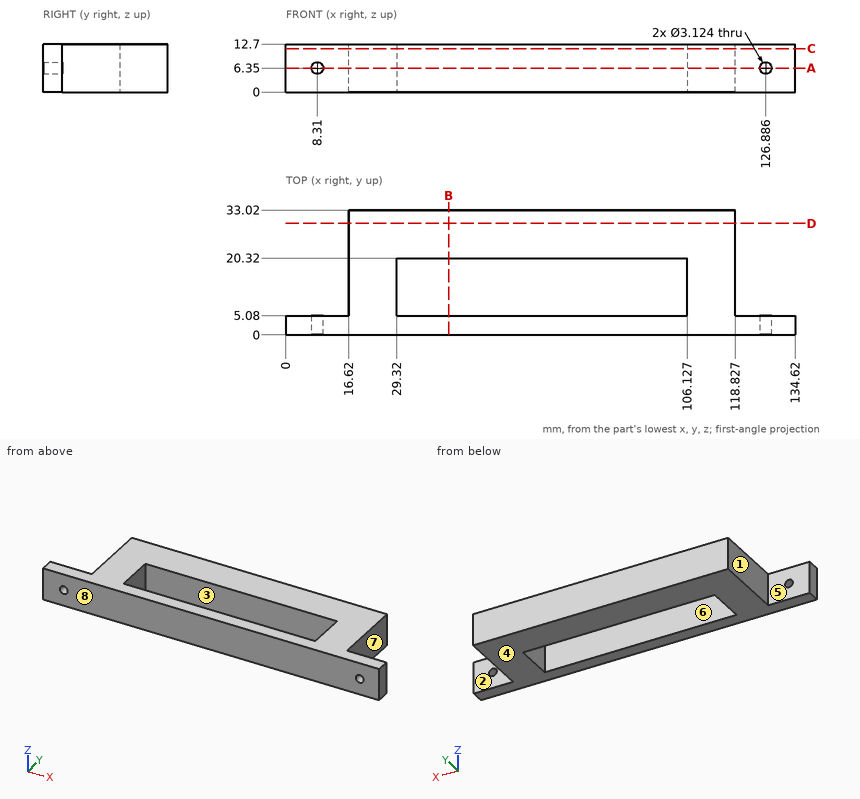
The figure shows three views and two pictorial views of one solid part (mm, origin at its lowest corner). Answer the questions. A direction names the side the tool comes from. Give positions to 0.01 mm unless a question says otherwise; leave off trailing zeros. Write each loop counter-clockwise with the first axis right and the second up, starting at its lowest first coordinate (ties: lowest second). Pieces come first, ordered by that corner, then holes. Notation, with made-up numbers: (69.5, 39.25) - (117.5, 39.25) arc R36 cw to (117.5, 75.25) - close; hole circle Ø2 at (-3.75, 76.25). An arc over 180 degrees is marked (long way). Return JSON: item names as keys, results as strings.
Q1. Consider line 1 along Y through (x, z) = (80.5, 10); line 2 along X through (y, z) = (7, 4.25); line 3 along X through (y, z) = (28.5, 4.5). Determine where each line is inside the solid, lowest interval first. Write a range as [from, to].
Reply:
{"line 1": "[0, 5.08], [20.32, 33.02]", "line 2": "[16.62, 29.32], [106.13, 118.83]", "line 3": "[16.62, 118.83]"}
Q2. A cutting plane is placed at D-D, the plane y = 29.5. Determine the outline of the cut face in (x, z), and give its area (3 significant figures).
Reply:
{"outline": "(16.62, 0) - (118.83, 0) - (118.83, 12.7) - (16.62, 12.7) - close", "area": "1,300 mm²"}
Q3. Given P1, Ø5, axis at y = 26, z = 2, coming from the +X side; P2, Ø1.9, axis at x = 126.89, z = 6.35, coming from the -Y side, each flat-ended and moving along its own axis, determine where each tip first touches the part or whether it passes through.
Reply:
{"P1": "x = 118.83", "P2": "through"}
Q4. A cutting plane is placed at B-B, the plane x = 43. Determine the outline of the cut face in (y, z).
Reply:
{"outline": "(0, 0) - (5.08, 0) - (5.08, 12.7) - (0, 12.7) - close; (20.32, 0) - (33.02, 0) - (33.02, 12.7) - (20.32, 12.7) - close"}
Q5. For the marked faces 1, 2, 3 and 4, determine the directions among +Z, -Z, +X, -X, +Y, -Y from which every point of the face is accessible in a straight line to the end or side of a thin tool.
Reply:
{"face 1": "+Z, -Z, -X, +Y", "face 2": "+Z, -Z, +X, +Y", "face 3": "+Z, -Z", "face 4": "-Z, +X, -X, +Y, -Y"}
Q6. For a pull along Y with two mould halves and no side action, classify the marked faces 5, 6, 7 and 8 as released by +Y, released by -Y, zero draft, split by the parting line, or undercut.
Reply:
{"face 5": "released by +Y", "face 6": "undercut", "face 7": "zero draft", "face 8": "released by -Y"}
Q7. A cutting plane is placed at A-A, the plane z = 6.35. Determine the outline of the cut face in (x, y), and give its area (3 significant figures).
Reply:
{"outline": "(0, 0) - (6.75, 0) - (6.75, 5.08) - (0, 5.08) - close; (9.87, 0) - (125.32, 0) - (125.32, 5.08) - (118.83, 5.08) - (118.83, 33.02) - (16.62, 33.02) - (16.62, 5.08) - (9.87, 5.08) - close; (128.45, 0) - (134.62, 0) - (134.62, 5.08) - (128.45, 5.08) - close; hole (29.32, 5.08) - (106.13, 5.08) - (106.13, 20.32) - (29.32, 20.32) - close", "area": "2,340 mm²"}
Q8. A cutting plane is placed at C-C, the plane z = 11.5. Determine the outline of the cut face in (x, y), and give its area (3 significant figures).
Reply:
{"outline": "(0, 0) - (134.62, 0) - (134.62, 5.08) - (118.83, 5.08) - (118.83, 33.02) - (16.62, 33.02) - (16.62, 5.08) - (0, 5.08) - close; hole (29.32, 5.08) - (106.13, 5.08) - (106.13, 20.32) - (29.32, 20.32) - close", "area": "2,370 mm²"}
